Answer from the drawing. Dimensions are ordinates in mm from the lowest x, y and z of the part. A direction names the side the tool comes from. Coordinates: 2 decimals unless noted, no trailing zeros. Order: outer loops, then holes, each group sorted by start corner. A loop starts at its lowest first (then second) coordinate and runs counter-clockwise, first axis right, second up. Notation, with made-up numbers: (-19.75, -4) -> (20.25, -4) arc R31 cw to (20.25, 23) -> close; hole circle Ø5 at (40.5, 40.25). An arc over 180 degrees is marked (long way). Answer as a JSON object with one key per item and string values. Group by question number.
1) Section C-C on z = 11 is taken. Determine the outline of the cut face in (x, y), and give its area (3 significant figures).
2) Section B-B on y = 40.5 is taken. Determine the outline of the cut face in (x, z), and give its area (4 significant figures).
3) Given pin 1 (6.5 mm diameter, centred on x = 40, z = 6, fed in from +Y); pin 2 (1.5 mm diameter, centred on x = 14, y = 43.5, fed in from +Z); pin 3 (3.5 mm diameter, centred on x = 35, y = 74, fed in from +Z), each flat-ended and moving along its own axis, determine where each tip first touches the part or whether it passes through.
4) A tool of negligible diameter and unlimited length cuts with its end or side. For the marked faces 1, 2, 3, 4 and 5, from which of +Z, -Z, +X, -X, +Y, -Y can it reach the whole face along a straight path? Write none if from no direction.
5) Section D-D on x = 35 is taken. Determine the outline of the cut face in (y, z).
6) Section A-A on z = 2 is taken. Determine the outline of the cut face in (x, y), and give its area (3 significant figures).
7) Consider L1, parallel to Y at x = 23.5, z = 17.5; L2, parallel to X at y = 20.5, z = 17.75; L3, parallel to X at y = 109, z = 11.25. Determine where each line is inside the solid, lowest interval first.
8) Determine the mould class of the marked faces 6, 7, 8 and 9 for opening direction X: released by +X, released by -X, zero draft, split by the parting line, or undercut.
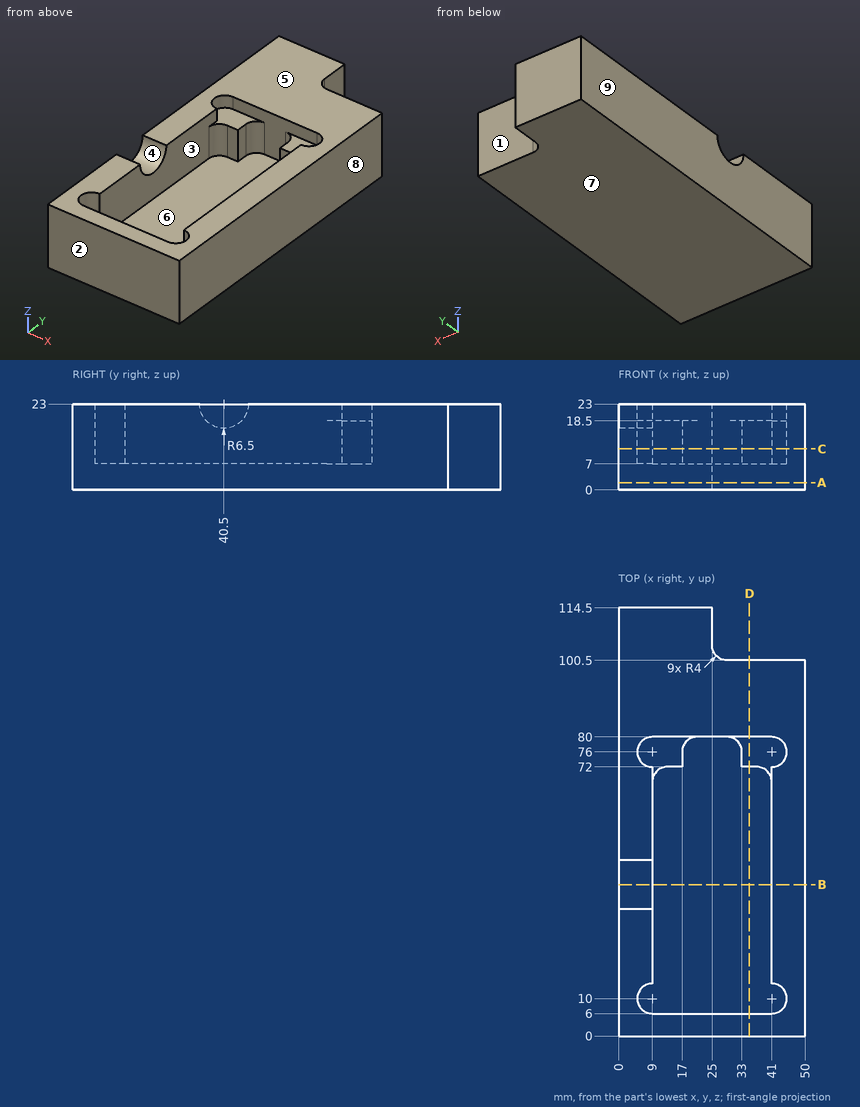
Worked answers:
{
 "1": {"outline": "(0, 0) -> (50, 0) -> (50, 100.5) -> (29, 100.5) arc R4 cw to (25, 104.5) -> (25, 114.5) -> (0, 114.5) -> close; hole (9, 6) -> (41, 6) arc R4 ccw to (41, 14) -> (41, 68) arc R4 ccw to (37, 72) -> (33, 72) -> (33, 76) arc R4 ccw to (29, 80) -> (21, 80) arc R4 ccw to (17, 76) -> (17, 72) -> (13, 72) arc R4 ccw to (9, 68) -> (9, 14) arc R4 ccw to start", "area": "3,100 mm²"},
 "2": {"outline": "(0, 0) -> (50, 0) -> (50, 23) -> (41, 23) -> (41, 7) -> (9, 7) -> (9, 16.5) -> (0, 16.5) -> close", "area": "579.5 mm²"},
 "3": {"pin 1": "stops at y = 100.5", "pin 2": "stops at z = 7", "pin 3": "stops at z = 18.5"},
 "4": {"face 1": "+Z, -Z, +X, +Y", "face 2": "+Z, -Z, +X, -X, -Y", "face 3": "+Z", "face 4": "+Z, -X", "face 5": "+Z, +X, -X, +Y, -Y"},
 "5": {"outline": "(0, 0) -> (100.5, 0) -> (100.5, 23) -> (80, 23) -> (80, 18.5) -> (72, 18.5) -> (72, 7) -> (6, 7) -> (6, 23) -> (0, 23) -> close"},
 "6": {"outline": "(0, 0) -> (50, 0) -> (50, 100.5) -> (29, 100.5) arc R4 cw to (25, 104.5) -> (25, 114.5) -> (0, 114.5) -> close", "area": "5,380 mm²"},
 "7": {"L1": "y = 0 to 6, 80 to 114.5", "L2": "x = 0 to 9, 41 to 50", "L3": "x = 0 to 25"},
 "8": {"face 6": "undercut", "face 7": "zero draft", "face 8": "released by +X", "face 9": "released by -X"}
}
